```python
from build123d import *

# Parameters (mm, degrees)
ESQUISSE1_W             = 11
ESQUISSE1_H             = 105
ESQUISSE1_R             = 3.2
BOSS_EXTRU_1_DEPTH      = 18.35
BOSS_EXTRU_1_2_DEPTH    = 18.35
ESQUISSE2_W             = 105
ESQUISSE2_H             = 105
BOSS_EXTRU_2_DEPTH      = 1.57
ESQUISSE3_W             = 105
ESQUISSE3_H             = 92
BOSS_EXTRU_3_DEPTH      = 45.54
ESQUISSE4_W             = 89
ESQUISSE4_H             = 7.4
BOSS_EXTRU_4_DEPTH      = 11.16
ENL_V_MAT_EXTRU_1_REACH = 136.411
ENL_V_MAT_EXTRU_2_REACH = 100.982
ESQUISSE7_W             = 5.75
ESQUISSE7_H             = 86
ESQUISSE8_W             = 27
ESQUISSE8_H             = 8
BOSS_EXTRU_5_DEPTH      = 7.1
ESQUISSE9_R             = 2.75
ESQUISSE9_R_2           = 1.25
ENL_V_MAT_EXTRU_3_DEPTH = 10
ENL_V_START             = -10
ENL_V_MAT_EXTRU_4_DEPTH = 10


with BuildPart() as part:
    # Esquisse1 → Boss.-Extru.1 (new body)
    with BuildSketch(Plane.XY):
        with Locations((-47, 0)):
            Rectangle(ESQUISSE1_W, ESQUISSE1_H)
        with Locations((-46, 46)):
            Circle(ESQUISSE1_R, mode=Mode.SUBTRACT)
        with Locations((-46, -33)):
            Circle(ESQUISSE1_R, mode=Mode.SUBTRACT)
    extrude(amount=BOSS_EXTRU_1_DEPTH)



with BuildPart() as body_2:
    # Esquisse1 → Boss.-Extru.1 2 (new body)
    with BuildSketch(Plane.XY):
        with Locations((47, 0)):
            Rectangle(ESQUISSE1_W, ESQUISSE1_H)
        with Locations((46, 46)):
            Circle(ESQUISSE1_R, mode=Mode.SUBTRACT)
        with Locations((46, -33)):
            Circle(ESQUISSE1_R, mode=Mode.SUBTRACT)
    extrude(amount=BOSS_EXTRU_1_2_DEPTH)


with BuildPart() as part_1:
    add(part.part)

    add(body_2.part)  # Boss.-Extru.2 merges body 2
    # Esquisse2 → Boss.-Extru.2 (add)
    with BuildSketch(Plane.XY.offset(18.35)):
        Rectangle(ESQUISSE2_W, ESQUISSE2_H)
    extrude(amount=BOSS_EXTRU_2_DEPTH)

    # Esquisse3 → Boss.-Extru.3 (add)
    with BuildSketch(Plane.XY.offset(19.92)):
        with Locations((0, 6.5)):
            Rectangle(ESQUISSE3_W, ESQUISSE3_H)
    extrude(amount=BOSS_EXTRU_3_DEPTH)

    # Esquisse4 → Boss.-Extru.4 (add)
    with BuildSketch(Plane.XY.offset(19.92)):
        with Locations((-3, -47.1)):
            Rectangle(ESQUISSE4_W, ESQUISSE4_H)
    extrude(amount=BOSS_EXTRU_4_DEPTH)

    # Esquisse6 → Enlèv. mat.-Extru.1 (cut, up to next)
    with BuildSketch(Plane(origin=(52.5, 0, 0), x_dir=(0, 0, -1), z_dir=(1, 0, 0)), mode=Mode.PRIVATE) as enl_v_mat_extru_1_sk1:
        Polygon((-62.46, -36.5), (-62.46, 49.5), (-39.24, 49.5), (-39.24, 46.81), (-59.94, 46.81), (-59.94, 45.71), (-39.24, 45.78), (-39.24, 43.09), (-59.94, 43.09), (-59.94, 41.99), (-39.24, 41.99), (-39.24, 39.3), (-59.94, 39.3), (-59.94, 38.2), (-39.24, 38.2), (-39.24, 35.51), (-59.94, 35.51), (-59.94, 34.41), (-39.24, 34.41), (-39.24, 31.72), (-59.94, 31.72), (-59.94, 30.62), (-39.24, 30.62), (-39.24, 27.93), (-59.94, 27.93), (-59.94, 26.83), (-39.24, 26.83), (-39.24, 24.14), (-59.94, 24.14), (-59.94, 23.04), (-39.24, 23.04), (-39.24, 20.35), (-59.94, 20.35), (-59.94, 19.25), (-39.24, 19.25), (-39.24, 16.56), (-59.94, 16.56), (-59.94, 15.46), (-39.24, 15.46), (-39.24, 12.77), (-59.94, 12.77), (-59.94, 11.67), (-39.24, 11.67), (-39.24, 8.98), (-59.94, 8.98), (-59.94, 7.88), (-39.24, 7.88), (-39.24, 5.19), (-59.94, 5.19), (-59.94, 4.09), (-39.24, 4.09), (-39.24, 1.4), (-59.94, 1.4), (-59.94, 0.3), (-39.24, 0.3), (-39.24, -2.39), (-59.94, -2.39), (-59.94, -3.49), (-39.24, -3.49), (-39.24, -6.18), (-59.94, -6.18), (-59.94, -7.28), (-39.24, -7.28), (-39.24, -9.97), (-59.94, -9.97), (-59.94, -11.07), (-39.24, -11.07), (-39.24, -13.76), (-59.94, -13.76), (-59.94, -14.86), (-39.24, -14.86), (-39.24, -17.55), (-59.94, -17.55), (-59.94, -18.65), (-39.24, -18.65), (-39.24, -21.34), (-59.94, -21.34), (-59.94, -22.44), (-39.24, -22.44), (-39.24, -25.13), (-59.94, -25.13), (-59.94, -26.23), (-39.24, -26.23), (-39.24, -28.92), (-59.94, -28.92), (-59.94, -30.02), (-39.24, -30.02), (-39.24, -32.71), (-59.94, -32.71), (-59.94, -33.81), (-39.24, -33.81), (-39.24, -36.5), align=None)
    enl_v_mat_extru_1_tool1 = extrude(enl_v_mat_extru_1_sk1.sketch, amount=-ENL_V_MAT_EXTRU_1_REACH, mode=Mode.PRIVATE) & part_1.part
    add(enl_v_mat_extru_1_tool1.solids().sort_by_distance((52.5, 6.508342, 51.269436))[0], mode=Mode.SUBTRACT)

    # Esquisse7 → Enlèv. mat.-Extru.2 (cut, up to next)
    with BuildSketch(Plane.XY.offset(65.46), mode=Mode.PRIVATE) as enl_v_mat_extru_2_sk1:
        with Locations((0.005, 6.5)):
            Rectangle(ESQUISSE7_W, ESQUISSE7_H)
    enl_v_mat_extru_2_tool1 = extrude(enl_v_mat_extru_2_sk1.sketch, amount=-ENL_V_MAT_EXTRU_2_REACH, mode=Mode.PRIVATE) & part_1.part
    # Esquisse7 → Enlèv. mat.-Extru.2 (cut, up to next)
    with BuildSketch(Plane.XY.offset(65.46), mode=Mode.PRIVATE) as enl_v_mat_extru_2_sk2:
        with Locations((-12.495, 6.5)):
            Rectangle(ESQUISSE7_W, ESQUISSE7_H)
    enl_v_mat_extru_2_tool2 = extrude(enl_v_mat_extru_2_sk2.sketch, amount=-ENL_V_MAT_EXTRU_2_REACH, mode=Mode.PRIVATE) & part_1.part
    # Esquisse7 → Enlèv. mat.-Extru.2 (cut, up to next)
    with BuildSketch(Plane.XY.offset(65.46), mode=Mode.PRIVATE) as enl_v_mat_extru_2_sk3:
        with Locations((-24.995, 6.5)):
            Rectangle(ESQUISSE7_W, ESQUISSE7_H)
    enl_v_mat_extru_2_tool3 = extrude(enl_v_mat_extru_2_sk3.sketch, amount=-ENL_V_MAT_EXTRU_2_REACH, mode=Mode.PRIVATE) & part_1.part
    # Esquisse7 → Enlèv. mat.-Extru.2 (cut, up to next)
    with BuildSketch(Plane.XY.offset(65.46), mode=Mode.PRIVATE) as enl_v_mat_extru_2_sk4:
        with Locations((25.005, 6.5)):
            Rectangle(ESQUISSE7_W, ESQUISSE7_H)
    enl_v_mat_extru_2_tool4 = extrude(enl_v_mat_extru_2_sk4.sketch, amount=-ENL_V_MAT_EXTRU_2_REACH, mode=Mode.PRIVATE) & part_1.part
    # Esquisse7 → Enlèv. mat.-Extru.2 (cut, up to next)
    with BuildSketch(Plane.XY.offset(65.46), mode=Mode.PRIVATE) as enl_v_mat_extru_2_sk5:
        with Locations((12.505, 6.5)):
            Rectangle(ESQUISSE7_W, ESQUISSE7_H)
    enl_v_mat_extru_2_tool5 = extrude(enl_v_mat_extru_2_sk5.sketch, amount=-ENL_V_MAT_EXTRU_2_REACH, mode=Mode.PRIVATE) & part_1.part
    add(enl_v_mat_extru_2_tool1.solids().sort_by_distance((0.005, 6.5, 65.46))[0], mode=Mode.SUBTRACT)
    add(enl_v_mat_extru_2_tool2.solids().sort_by_distance((-12.495, 6.5, 65.46))[0], mode=Mode.SUBTRACT)
    add(enl_v_mat_extru_2_tool3.solids().sort_by_distance((-24.995, 6.5, 65.46))[0], mode=Mode.SUBTRACT)
    add(enl_v_mat_extru_2_tool4.solids().sort_by_distance((25.005, 6.5, 65.46))[0], mode=Mode.SUBTRACT)
    add(enl_v_mat_extru_2_tool5.solids().sort_by_distance((12.505, 6.5, 65.46))[0], mode=Mode.SUBTRACT)

    # Esquisse8 → Boss.-Extru.5 (add)
    with BuildSketch(Plane(origin=(0, 0, 18.35), x_dir=(-1, 0, 0), z_dir=(0, 0, -1))):
        with Locations((-27, 47.5)):
            Rectangle(ESQUISSE8_W, ESQUISSE8_H)
    extrude(amount=BOSS_EXTRU_5_DEPTH)

    # Esquisse9 → Enlèv. mat.-Extru.3 (cut)
    # profile 1 of 4: a face of its own
    with BuildSketch(Plane.ZY.offset(52.5)):
        with Locations((13.25, 36.1)):
            Circle(ESQUISSE9_R)
        with Locations((13.25, 36.1)):
            Circle(ESQUISSE9_R_2, mode=Mode.SUBTRACT)
    # profile 2 of 4: a face of its own
    with BuildSketch(Plane.ZY.offset(52.5)):
        Polygon((18.85, 26.5), (18.85, 22.626049106), (20.53, 22.626049106), (20.53, 18.373950894), (18.85, 18.373950894), (18.85, 14.5), (12, 14.5), (12, 26.5), align=None)
    # profile 3 of 4: a face of its own
    with BuildSketch(Plane.ZY.offset(52.5)):
        with BuildLine():
            Line((20.25, 37.6), (20.25, 34.6))
            ThreePointArc((20.25, 34.6), (19.25, 33.6), (18.25, 34.6))
            Line((18.25, 34.6), (18.25, 37.6))
            ThreePointArc((18.25, 37.6), (19.25, 38.6), (20.25, 37.6))
        make_face()
    # profile 4 of 4: a face of its own
    with BuildSketch(Plane.ZY.offset(52.5)):
        Polygon((18.85, -13.5), (18.85, -27.5), (16.85, -27.5), (16.85, -26.5), (14.85, -23), (14.85, -18), (16.85, -14.5), (16.85, -13.5), align=None)
    extrude(amount=-ENL_V_MAT_EXTRU_3_DEPTH, mode=Mode.SUBTRACT)

    # Esquisse10 → Enlèv. mat.-Extru.4 (cut)
    with BuildSketch(Plane(origin=(52.5, 0, 0), x_dir=(0, 0, -1), z_dir=(1, 0, 0)).offset(ENL_V_START)):
        with BuildLine():
            Line((-20.25, 34.6), (-20.25, 37.6))
            ThreePointArc((-20.25, 37.6), (-19.25, 38.6), (-18.25, 37.6))
            Line((-18.25, 37.6), (-18.25, 34.6))
            ThreePointArc((-18.25, 34.6), (-19.25, 33.6), (-20.25, 34.6))
        make_face()
    extrude(amount=ENL_V_MAT_EXTRU_4_DEPTH, mode=Mode.SUBTRACT)


solid = part_1.part
```
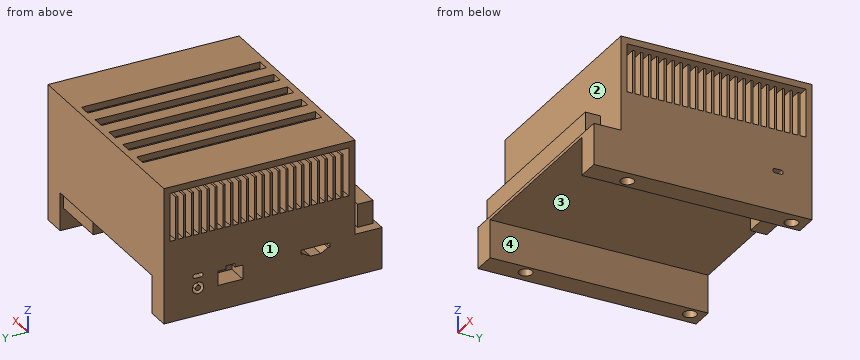
Here's how the part is built. I have some questions about the finished solid (model axes, mm). Face numbers are marked on the shaded views. Give positions to 0.01 mm unless a question says otherwise; leave off trailing zeros. Order: outer loops, then holes, each group sorted by start corner. A loop starts at its lowest first (then second) coordinate and runs counter-clockwise, first axis right, second up. Notation, with made-up numbers: (65, 1) - (104, 1) arc R29 ccw to (104, 24) - close; hole circle Ø10 at (61, 38.25). An arc over 180 degrees is marked (long way). Answer as a JSON object with one key per item and string values. Group by question number.
Item 1: If we mould it in two halves opening along X, with no side actions, what happens to the marked faces 1, 2, 3 and 4? For each: pulls with the +X half, pulls with the -X half, needs draft (parallel to the pull), parting line crosses it, or undercut.
Item 2: If we section it at A-A on z = 4.5: Please give me the cut outline in (x, y).
Item 3: If we section it at B-B on x = 46: Give the number of separate pieces and of enclosed holes in the cut face, and give its area (3 significant figures).
Item 4: Please list where these lines run through material, in increasing order: probe 1 along Y at (x, z) = (-46, 13); probe 2 along Y at (x, z) = (46, 5.5); probe 3 along Z at (x, y) = (-35, 25).
Item 5: For P1, Ø5.5, axis at x = 4, z = 23.5, coming from the -Y side; P2, Ø4, axis at x = 39, y = 33, coming from the -Z side; P3, Ø1.3, axis at x = 2, y = -27, coming from the +Z side, each with a flat end and sliding along its axis, tell me the tip position at first contact or that it passes through.
Item 6: If we section it at C-C on z = 33.5: Please give me the cut outline in (x, y), and give its area (3 significant figures).
Result set:
{
 "1": {"face 1": "pulls with the -X half", "face 2": "needs draft", "face 3": "undercut", "face 4": "undercut"},
 "2": {"outline": "(-52.5, -52.5) - (-41.5, -52.5) - (-41.5, 52.5) - (-52.5, 52.5) - close; (41.5, -52.5) - (52.5, -52.5) - (52.5, 52.5) - (41.5, 52.5) - close; hole circle Ø6.4 at (-46, -33); hole circle Ø6.4 at (-46, 46); hole circle Ø6.4 at (46, -33); hole circle Ø6.4 at (46, 46)"},
 "3": {"separate pieces": "1", "enclosed holes": "2", "area": "4,540 mm²"},
 "4": {"probe 1": "-52.5 to -36.2, -29.8 to 14.5, 26.5 to 33.36, 34.88 to 37.32, 38.84 to 42.8, 49.2 to 52.5", "probe 2": "-52.5 to -36.2, -29.8 to 42.8, 49.2 to 52.5", "probe 3": "18.35 to 39.24, 62.46 to 65.46"},
 "5": {"P1": "y = -50.8", "P2": "z = 18.35", "P3": "z = 39.24"},
 "6": {"outline": "(-52.5, -39.5) - (52.5, -39.5) - (52.5, 52.5) - (-52.5, 52.5) - close", "area": "9,660 mm²"}
}
